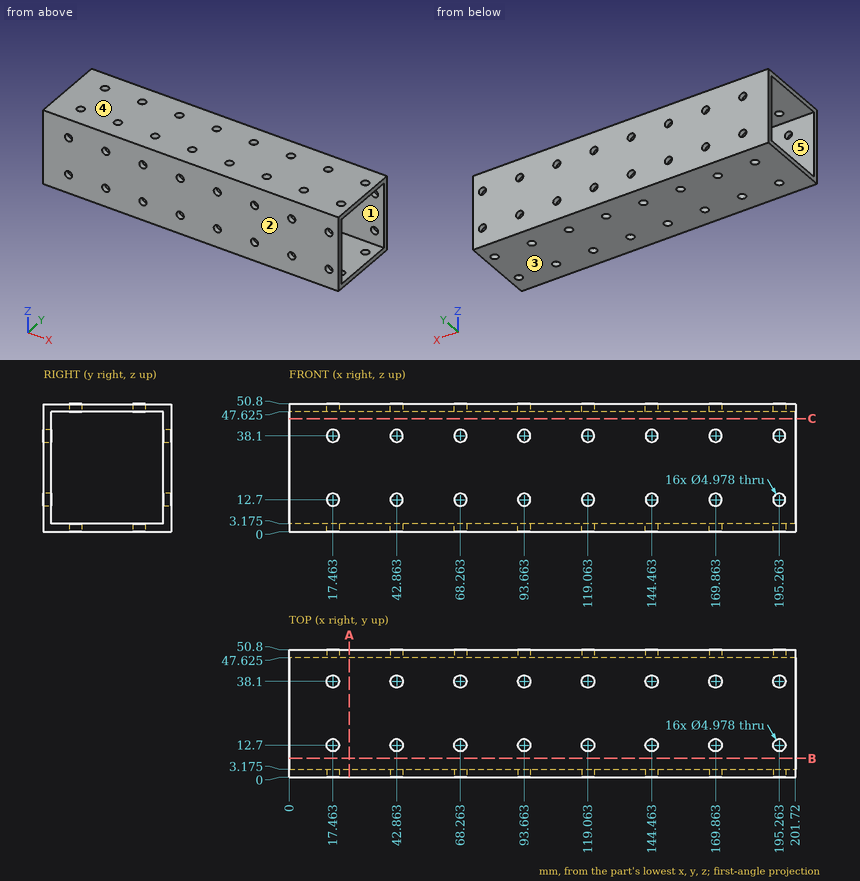
Here's the drawing with two shaded views (mm, measured from the low corner). I have some questions. A direction names the side the tool comes from. Give positions to 0.01 mm unless a question says otherwise; leave off trailing zeros. Order: outer loops, then holes, each group sorted by start corner. A loop starts at its lowest first (then second) coordinate and runs counter-clockwise, first axis right, second up. Notation, with made-up numbers: (49.5, 47) -> (94.5, 47) arc R20 cw to (94.5, 67) -> close; hole circle Ø7 at (66, 78.5). An arc over 180 degrees is marked (long way). Use a Markdown table: item, result. Add a question column.
Item 1: I need wall thicknesses on line 1 (Y direction, x = 130, z = 14.5) (1 decimal). Which ranges of the line are inside material? Lowest first, please.
Item 2: For the marked faces 4 and 5, which set-ups out of +Z, -Z, +X, -X, +Y, -Y let a thin tool reach every point of the face, with its end or its side?
Item 3: Imagine slicing it at A-A on x = 24. Please give me the cut outline in (y, z) (1 decimal).
Item 4: Imagine slicing it at B-B on y = 7.5. Please give me the cut outline in (x, z) (1 decimal), plus the area to 3 significant figures.
Item 5: If we mould it in two halves opening along Z, with no side actions, what happens to the marked faces 1, 2 and 3? For each: pulls with the +Z half, pulls with the -Z half, needs draft (parallel to the pull), parting line crosses it, or undercut.
Data:
| question | item | result |
|---|---|---|
| 1 | line 1 | y = 0 to 3.2, 47.6 to 50.8 |
| 2 | face 4 | +Z, +X, -X, +Y, -Y |
| 2 | face 5 | +X, -X |
| 3 | outline | (0, 0) -> (50.8, 0) -> (50.8, 50.8) -> (0, 50.8) -> close; hole (3.2, 3.2) -> (47.6, 3.2) -> (47.6, 47.6) -> (3.2, 47.6) -> close |
| 4 | outline | (0, 0) -> (201.7, 0) -> (201.7, 3.2) -> (0, 3.2) -> close; (0, 47.6) -> (201.7, 47.6) -> (201.7, 50.8) -> (0, 50.8) -> close |
| 4 | area | 1,280 mm² |
| 5 | face 1 | undercut |
| 5 | face 2 | needs draft |
| 5 | face 3 | pulls with the -Z half |
